Work out the finished part from the listing and answer in its coordinate system (mm). Face numbers are marked on the shaded views. A direction names the side the tool comes from. Give positions to 0.01 mm unless a question says otherwise; leave off trailing zeros. Loops run counter-clockwise (first coordinate to the right, second up) from the corner with the lowest first, then second, coordinate; pieces in that order, holes last.
from build123d import *

# Parameters (mm, degrees)
DODANIE_WYCI_GNI_CIE1_DEPTH = 1.6
SZKIC2_3_R                  = 2
WYTNIJ_WYCI_GNI_CIE1_DEPTH  = 1.6
SZKIC3_W                    = 11.2
SZKIC3_H                    = 4
DODANIE_WYCI_GNI_CIE2_DEPTH = 3.9


with BuildPart() as part:
    # Szkic2 → Dodanie-wyci_gni_cie1 (new body)
    with BuildSketch(Plane(origin=(0, 0, 0), x_dir=(1, 0, 0), z_dir=(0, 1, 0))):
        with BuildLine():
            Line((-10, -21), (-10, -21.5))
            ThreePointArc((-10, -21.5), (-9.707106781, -22.207106781), (-9, -22.5))
            Line((-9, -22.5), (9, -22.5))
            ThreePointArc((9, -22.5), (9.707106781, -22.207106781), (10, -21.5))
            Line((10, -21.5), (10, -21))
            Line((10, -21), (18, -21))
            ThreePointArc((18, -21), (20.121320344, -20.121320344), (21, -18))
            Line((21, -18), (21, 18))
            ThreePointArc((21, 18), (20.121320344, 20.121320344), (18, 21))
            Line((18, 21), (-18, 21))
            ThreePointArc((-18, 21), (-20.121320344, 20.121320344), (-21, 18))
            Line((-21, 18), (-21, -18))
            ThreePointArc((-21, -18), (-20.121320344, -20.121320344), (-18, -21))
            Line((-18, -21), (-10, -21))
        make_face()
    extrude(amount=DODANIE_WYCI_GNI_CIE1_DEPTH)

    # Szkic2_3 → Wytnij-wyci_gni_cie1 (cut)
    with BuildSketch(Plane(origin=(0, 0, 0), x_dir=(1, 0, 0), z_dir=(0, 1, 0))):
        with Locations((15.696699141, 15.696699141)):
            Circle(SZKIC2_3_R)
        with Locations((-15.696699141, 15.696699141)):
            Circle(SZKIC2_3_R)
        with Locations((15.696699141, -15.696699141)):
            Circle(SZKIC2_3_R)
        with Locations((-15.696699141, -15.696699141)):
            Circle(SZKIC2_3_R)
    extrude(amount=WYTNIJ_WYCI_GNI_CIE1_DEPTH, mode=Mode.SUBTRACT)

    # Szkic3 → Dodanie-wyci_gni_cie2 (add)
    with BuildSketch(Plane(origin=(0, 1.6, 0), x_dir=(1, 0, 0), z_dir=(0, 1, 0))):
        with Locations((0, 15.8)):
            Rectangle(SZKIC3_W, SZKIC3_H)
    extrude(amount=DODANIE_WYCI_GNI_CIE2_DEPTH)


solid = part.part
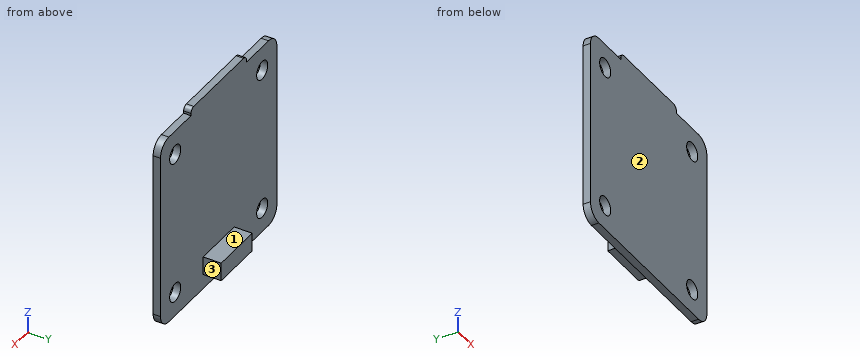
Item 1: Find section A-A, the plane x = 17. Write down the section's boundary in (y, z), plus the area to 3 significant figures.
Item 2: Find section D-D, the plane z = 4.5. Write down the section's boundary in (x, y), plus the area to 3 significant figures.
Item 3: Flat-ended cylindrical pins translate along their axes: pin 1 Ø0.5 at (x, y) = (-15, 1) entering from +Z; pin 2 Ø4.5 at (x, z) = (15.7, 15.7) entering from +Y; pin 3 Ø2 at (y, z) = (4, -15) entering from +X. Find the tip coordinate at first contact, or state that the pin passes through.
Item 4: For the marked faces 1, 2 and 3, determine the directions among +Z, -Z, +X, -X, +Y, -Y from which every point of the face is accessible in a straight line to the end or side of a thin tool.
Item 5: Find section C-C, the plane y = 2.4. Write down the section's boundary in (x, z), plus the area to 3 significant figures.
Item 6: Consider line 1 (Y direction, x = 19, z = 0); line 2 (Z direction, x = -1, y = 4.1); line 3 (X direction, y = 3.7, z = -15). Determine where each line is inside the solid, lowest interval first.
Item 7: Find section B-B, the plane x = 5. Write down the section's boundary in (y, z).
Ans:
1. outline: (0, -21) - (1.6, -21) - (1.6, -17.21) - (0, -17.21) - close; (0, -14.18) - (1.6, -14.18) - (1.6, 14.18) - (0, 14.18) - close; (0, 17.21) - (1.6, 17.21) - (1.6, 21) - (0, 21) - close
1. area: 57.5 mm2
2. outline: (-21, 0) - (21, 0) - (21, 1.6) - (-21, 1.6) - close
2. area: 67.2 mm2
3. pin 1: stops at z = 21
3. pin 2: stops at y = 1.6
3. pin 3: stops at x = 5.6
4. face 1: +Z, +X, -X, +Y
4. face 2: +Z, -Z, +X, -X, -Y
4. face 3: +Z, -Z, +X, +Y
5. outline: (-5.6, -17.8) - (5.6, -17.8) - (5.6, -13.8) - (-5.6, -13.8) - close
5. area: 44.8 mm2
6. line 1: y = 0 to 1.6
6. line 2: z = -17.8 to -13.8
6. line 3: x = -5.6 to 5.6
7. outline: (0, -21) - (1.6, -21) - (1.6, -17.8) - (5.5, -17.8) - (5.5, -13.8) - (1.6, -13.8) - (1.6, 22.5) - (0, 22.5) - close
